Read the model definition and answer for the solid it produces. Units are mm, in the model's axes. A direction names the side the tool comes from. Round coordinates to 2 decimals unless told otherwise and drop trailing zeros. Order: outer loops, then holes, each group sorted by start corner. A loop starts at its lowest first (then second) coordinate and runs counter-clockwise, first axis right, second up. Notation, with made-up numbers: (69.5, 19.25) - (111.5, 19.25) arc R21 cw to (111.5, 50.25) - close; hole circle Ø4 at (60, -20.5). An arc over 180 degrees is marked (long way). One line per question, with ' | ' between items. Start each with the question number.
1) The part is cut by section D-D, the plane z = -11.5. Give the vertices of the cut face in (x, y), plus the area to 3 significant figures.
2) For faces 3 (the flat face through (0, 6, 7)), 4 (the flat face through (12.154, 7, 0)), determine the directions among +Z, -Z, +X, -X, +Y, -Y from which every point of the face is accessible in a straight line to the end or side of a thin tool.
3) Straight lines are drawn through the part: line 1 (X direction, y = 6.75, z = 0.25); line 2 (Y direction, x = 1.75, z = -13.5); line 3 (X direction, y = 8, z = 7). For each, find the intervals that lie inside material, in ascending order. Write a range as from..to.
4) The mould has two halves that part along Z. Classify faces 1 (the cylindrical face through (0.66, 7.232, -14.985)), 2 (the flat face through (10.63, 7.27, 2.61)): pulls with the +Z half, pulls with the -Z half, needs draft (parallel to the pull), parting line crosses it, or undercut.
5) The part is cut by section C-C, the plane y = 6.5. Give the vertices of the cut face in (x, z).
6) The part is cut by section A-A, the plane x = 0. Give the vertices of the cut face in (y, z).
7) Flat-ended cylindrical pins translate along their axes: pin 1 (2 mm diameter, centred on x = -1.5, y = 7, fed in from -Z); pin 2 (1 mm diameter, centred on x = 2.5, y = 6, fed in from +Z); pin 3 (5 mm diameter, centred on x = 3.5, y = 4, fed in from -Z). Find the tip coordinate at first contact, or state that the pin passes through.
8) The part is cut by section B-B, the plane z = 0. Give the vertices of the cut face in (x, y).
from build123d import *

# Parameters (mm, degrees)
CROQUIS1_R              = 8.5
SALIENTE_EXTRUIR1_DEPTH = 2
CROQUIS2_R              = 7.5
SALIENTE_EXTRUIR2_DEPTH = 4
CROQUIS3_R              = 15
SALIENTE_EXTRUIR3_DEPTH = 2.5
REDONDEO1_R             = 3
CORTAR_EXTRUIR1_DEPTH   = 2.5


with BuildPart() as part:
    # Croquis1 → Saliente-Extruir1 (new body)
    with BuildSketch(Plane(origin=(0, 0, 0), x_dir=(1, 0, 0), z_dir=(0, 1, 0))):
        with Locations(Location((0, 0, 0), (0, 0, 270))):
            Circle(CROQUIS1_R)
    extrude(amount=SALIENTE_EXTRUIR1_DEPTH)

    # Croquis2 → Saliente-Extruir2 (add)
    with BuildSketch(Plane(origin=(0, 2, 0), x_dir=(1, 0, 0), z_dir=(0, 1, 0))):
        with Locations(Location((0, 0, 0), (0, 0, 270))):
            Circle(CROQUIS2_R)
    extrude(amount=SALIENTE_EXTRUIR2_DEPTH)

    # Croquis3 → Saliente-Extruir3 (add)
    with BuildSketch(Plane(origin=(0, 6, 0), x_dir=(1, 0, 0), z_dir=(0, 1, 0))):
        with Locations(Location((0, 0, 0), (0, 0, 270))):
            Circle(CROQUIS3_R)
    extrude(amount=SALIENTE_EXTRUIR3_DEPTH)

    # Redondeo1
    # the kernel refuses this fillet: 3 mm, written as the material it takes off along each edge
    with BuildSketch(Plane(origin=(0, 0, 0), x_dir=(0, 0, 1), z_dir=(-1, 0, 0))) as redondeo1_piece_1:
        with BuildLine():
            CenterArc((5.671572875, 3), REDONDEO1_R, 270, 70.528779366)
            Line((5.671572875, 0), (5.671572875, -0.06))
            Line((5.671572875, -0.06), (8.5, -0.06))
            Line((8.5, -0.06), (8.56, 0))
            ThreePointArc((8.56, 0), (8.56, 1), (8.556568542, 1.98))
            Line((8.556568542, 1.98), (8.5, 2))
        make_face()
    revolve(axis=Axis((0, 0, 0), (0, 1, 0)), mode=Mode.SUBTRACT)

    # Croquis4 → Cortar-Extruir1 (cut)
    with BuildSketch(Plane(origin=(0, 8.5, 0), x_dir=(1, 0, 0), z_dir=(0, 1, 0))):
        Polygon((12.154001459, -1.732050808), (12.154001459, 1.732050808), (9.154001459, 3.464101615), (6.154001459, 1.732050808), (6.154001459, -1.732050808), (9.154001459, -3.464101615), align=None)
        Polygon((3.464101615, 9.154001459), (1.732050808, 12.154001459), (-1.732050808, 12.154001459), (-3.464101615, 9.154001459), (-1.732050808, 6.154001459), (1.732050808, 6.154001459), align=None)
        Polygon((-1.732050808, -12.154001459), (1.732050808, -12.154001459), (3.464101615, -9.154001459), (1.732050808, -6.154001459), (-1.732050808, -6.154001459), (-3.464101615, -9.154001459), align=None)
        Polygon((-12.154001459, 1.732050808), (-12.154001459, -1.732050808), (-9.154001459, -3.464101615), (-6.154001459, -1.732050808), (-6.154001459, 1.732050808), (-9.154001459, 3.464101615), align=None)
    extrude(amount=-CORTAR_EXTRUIR1_DEPTH, mode=Mode.SUBTRACT)


solid = part.part
Values:
1) outline: (-9.63, 6) - (-2.11, 6) - (-2.11, 8.5) - (-9.63, 8.5) - close; (2.11, 6) - (9.63, 6) - (9.63, 8.5) - (2.11, 8.5) - close | area: 37.6 mm^2
2) face 3: +Y | face 4: +Y, -Y
3) line 1: x = -15..-12.15, -6.15..6.15, 12.15..15 | line 2: y = 6..8.5 | line 3: x = -13.27..-2.22, 2.22..13.27
4) face 1: parting line crosses it | face 2: undercut
5) outline: circle Ø30 at (0, 0); hole (-12.15, -1.73) - (-9.15, -3.46) - (-6.15, -1.73) - (-6.15, 1.73) - (-9.15, 3.46) - (-12.15, 1.73) - close; hole (-3.46, -9.15) - (-1.73, -12.15) - (1.73, -12.15) - (3.46, -9.15) - (1.73, -6.15) - (-1.73, -6.15) - close; hole (-3.46, 9.15) - (-1.73, 6.15) - (1.73, 6.15) - (3.46, 9.15) - (1.73, 12.15) - (-1.73, 12.15) - close; hole (6.15, -1.73) - (9.15, -3.46) - (12.15, -1.73) - (12.15, 1.73) - (9.15, 3.46) - (6.15, 1.73) - close
6) outline: (0, -5.67) arc R3 ccw to (2, -8.5) - (2, -7.5) - (6, -7.5) - (6, -6.15) - (8.5, -6.15) - (8.5, 6.15) - (6, 6.15) - (6, 7.5) - (2, 7.5) - (2, 8.5) arc R3 ccw to (0, 5.67) - close; (6, -15) - (8.5, -15) - (8.5, -12.15) - (6, -12.15) - close; (6, 12.15) - (8.5, 12.15) - (8.5, 15) - (6, 15) - close
7) pin 1: stops at z = -14.99 | pin 2: stops at z = 14.87 | pin 3: stops at z = -14.87
8) outline: (-15, 6) - (-12.15, 6) - (-12.15, 8.5) - (-15, 8.5) - close; (-8.5, 2) arc R3 ccw to (-5.67, 0) - (5.67, 0) arc R3 ccw to (8.5, 2) - (7.5, 2) - (7.5, 6) - (6.15, 6) - (6.15, 8.5) - (-6.15, 8.5) - (-6.15, 6) - (-7.5, 6) - (-7.5, 2) - close; (12.15, 6) - (15, 6) - (15, 8.5) - (12.15, 8.5) - close
